```python
from build123d import *

# Parameters (mm, degrees)
SKETCH1_W           = 22
SKETCH1_H           = 47
SKETCH1_W_2         = 11
SKETCH1_H_2         = 11
BOSS_EXTRUDE_DEPTH  = 3
SKETCH5_W           = 1.8
SKETCH5_H           = 47
BOSS_EXTRUDE1_DEPTH = 2


with BuildPart() as part:
    # Sketch1 → Boss-Extrude (new body)
    with BuildSketch(Plane(origin=(0, 0, 0), x_dir=(1, 0, 0), z_dir=(0, 1, 0))):
        Rectangle(SKETCH1_W, SKETCH1_H)
        with Locations((0, 12)):
            Rectangle(SKETCH1_W_2, SKETCH1_H_2, mode=Mode.SUBTRACT)
    extrude(amount=BOSS_EXTRUDE_DEPTH)

    # Sketch5 → Boss-Extrude1 (add)
    with BuildSketch(Plane(origin=(0, 3, 0), x_dir=(1, 0, 0), z_dir=(0, 1, 0))):
        with Locations((-7.9, 0)):
            Rectangle(SKETCH5_W, SKETCH5_H)
        with Locations((7.9, 0)):
            Rectangle(SKETCH5_W, SKETCH5_H)
    extrude(amount=BOSS_EXTRUDE1_DEPTH)


solid = part.part
```
The listing builds one solid part. Answer for the finished solid, in the listing's coordinates (mm). A direction names the side the tool comes from. Coordinates: 2 decimals unless noted, no trailing zeros. Loops run counter-clockwise (first coordinate to the right, second up) from the corner with the lowest first, then second, coordinate; pieces in that order, holes last. Notation, with made-up numbers: (4, 5.5) -> (58, 5.5) arc R33 cw to (58, 36.5) -> close; hole circle Ø10 at (84.5, -38). An arc over 180 degrees is marked (long way). Use one line per item in the form item = value. Start each with the question number.
Item 1: The part is cut by section D-D on z = 19.5. Determine the outline of the cut face in (x, y).
Item 2: A tool of negligible diameter and unlimited length cuts with its end or side. For faces 1 (the face through (0, 1, -17.5)), 2 (the face through (-7, 4, 0)), 3 (the face through (8.8, 4, 0)), from which of +Z, -Z, +X, -X, +Y, -Y can it reach the whole face along a straight path? Write none if from no direction.
Item 3: The mould has two halves that part along X. Classify faces 4 (the face through (-11, 1, 0)), 5 (the face through (10, 3, 0)), 6 (the face through (0, 1, -6.5)): released by +X, released by -X, zero draft, split by the parting line, or undercut.
Item 4: The part is cut by section C-C on z = -9. Determine the outline of the cut face in (x, y), then the cut area to 3 significant figures.
Item 5: Flat-ended cylindrical pins translate along their axes: pin 1 Ø0.7 at (x, z) = (10.5, 10.5) entering from +Y; pin 2 Ø0.6 at (y, z) = (3.5, 9.5) entering from +X; pin 3 Ø1.6 at (y, z) = (4, 6.5) entering from -X; pin 4 Ø8 at (x, z) = (6, -9.5) entering from -Y. Find the tip coordinate at first contact, or state that the pin passes through.
Item 6: The part is cut by section B-B on y = 4.15. Determine the outline of the cut face in (x, z).
Item 7: Consider L1, parallel to X at y = 4, z = -1; L2, parallel to X at y = 1.1, z = -14; L3, parallel to Z at x = -0.25, y = 2.5. Determine where each line is inside the solid, lowest interval first. Write a range as [from, to].
Item 8: The part is cut by section A-A on x = -1.5. Determine the outline of the cut face in (y, z).
Answer key:
q1.outline = (-11, 0) -> (11, 0) -> (11, 3) -> (8.8, 3) -> (8.8, 5) -> (7, 5) -> (7, 3) -> (-7, 3) -> (-7, 5) -> (-8.8, 5) -> (-8.8, 3) -> (-11, 3) -> close
q2.face_1 = +Y, -Y
q2.face_2 = +Z, -Z, +Y
q2.face_3 = +Z, -Z, +X, +Y
q3.face_4 = released by -X
q3.face_5 = zero draft
q3.face_6 = undercut
q4.outline = (-11, 0) -> (-5.5, 0) -> (-5.5, 3) -> (-7, 3) -> (-7, 5) -> (-8.8, 5) -> (-8.8, 3) -> (-11, 3) -> close; (5.5, 0) -> (11, 0) -> (11, 3) -> (8.8, 3) -> (8.8, 5) -> (7, 5) -> (7, 3) -> (5.5, 3) -> close
q4.area = 40.2 mm2
q5.pin_1 = 3
q5.pin_2 = 8.8
q5.pin_3 = -8.8
q5.pin_4 = 0
q6.outline = (-8.8, -23.5) -> (-7, -23.5) -> (-7, 23.5) -> (-8.8, 23.5) -> close; (7, -23.5) -> (8.8, -23.5) -> (8.8, 23.5) -> (7, 23.5) -> close
q7.L1 = [-8.8, -7], [7, 8.8]
q7.L2 = [-11, -5.5], [5.5, 11]
q7.L3 = [-23.5, -17.5], [-6.5, 23.5]
q8.outline = (0, -23.5) -> (3, -23.5) -> (3, -17.5) -> (0, -17.5) -> close; (0, -6.5) -> (3, -6.5) -> (3, 23.5) -> (0, 23.5) -> close
